from build123d import *

# Parameters (mm, degrees)
BOSS_EXTRUDE1_DEPTH = 1
SKETCH3_R           = 1.2
SKETCH3_R_2         = 3.05
CUT_EXTRUDE1_DEPTH  = 54.01311748


with BuildPart() as part:
    # Sketch1 → Boss-Extrude1 (new, symmetric)
    with BuildSketch(Plane(origin=(0, 0, 0), x_dir=(1, 0, 0), z_dir=(0, 1, 0))):
        with BuildLine():
            Line((22.2, 8.95), (22.2, -8.95))
            Line((22.2, -8.95), (40.625, -8.95))
            Line((40.625, -8.95), (40.625, -25.15))
            Line((40.625, -25.15), (22.879630679, -25.15))
            ThreePointArc((22.879630679, -25.15), (0, -34), (-22.879630679, -25.15))
            Line((-22.879630679, -25.15), (-40.625, -25.15))
            Line((-40.625, -25.15), (-40.625, -8.95))
            Line((-40.625, -8.95), (-22.2, -8.95))
            Line((-22.2, -8.95), (-22.2, 8.95))
            Line((-22.2, 8.95), (-40.625, 8.95))
            Line((-40.625, 8.95), (-40.625, 25.15))
            Line((-40.625, 25.15), (-22.879630679, 25.15))
            ThreePointArc((-22.879630679, 25.15), (0, 34), (22.879630679, 25.15))
            Line((22.879630679, 25.15), (40.625, 25.15))
            Line((40.625, 25.15), (40.625, 8.95))
            Line((40.625, 8.95), (22.2, 8.95))
        make_face()
    extrude(amount=BOSS_EXTRUDE1_DEPTH, both=True)

    # Sketch3 → Cut-Extrude1 (cut, through all)
    with BuildSketch(Plane(origin=(0, 1, 0), x_dir=(1, 0, 0), z_dir=(0, 1, 0))):
        with Locations(Location((-36.95, 17.05, 0), (0, 0, 270))):
            Circle(SKETCH3_R)
        with Locations(Location((-30, 17.05, 0), (0, 0, 270))):
            Circle(SKETCH3_R_2)
        with Locations(Location((-23.05, 17.05, 0), (0, 0, 270))):
            Circle(SKETCH3_R)
        with Locations(Location((23.05, 17.05, 0), (0, 0, 90))):
            Circle(SKETCH3_R)
        with Locations(Location((30, 17.05, 0), (0, 0, 90))):
            Circle(SKETCH3_R_2)
        with Locations(Location((36.95, 17.05, 0), (0, 0, 90))):
            Circle(SKETCH3_R)
        with Locations(Location((36.95, -17.05, 0), (0, 0, 270))):
            Circle(SKETCH3_R)
        with Locations(Location((30, -17.05, 0), (0, 0, 270))):
            Circle(SKETCH3_R_2)
        with Locations(Location((23.05, -17.05, 0), (0, 0, 270))):
            Circle(SKETCH3_R)
        with Locations(Location((-23.05, -17.05, 0), (0, 0, 90))):
            Circle(SKETCH3_R)
        with Locations(Location((-30, -17.05, 0), (0, 0, 90))):
            Circle(SKETCH3_R_2)
        with Locations(Location((-36.95, -17.05, 0), (0, 0, 90))):
            Circle(SKETCH3_R)
        with BuildLine():
            Line((1.55, 27.775), (1.55, -27.775))
            ThreePointArc((1.55, -27.775), (0, -29.325), (-1.55, -27.775))
            Line((-1.55, -27.775), (-1.55, 27.775))
            ThreePointArc((-1.55, 27.775), (0, 29.325), (1.55, 27.775))
        make_face()
        with BuildLine():
            Line((-18.5, 1.55), (-6.05, 1.55))
            ThreePointArc((-6.05, 1.55), (-4.5, 0), (-6.05, -1.55))
            Line((-6.05, -1.55), (-18.5, -1.55))
            ThreePointArc((-18.5, -1.55), (-20.05, 0), (-18.5, 1.55))
        make_face()
        with BuildLine():
            Line((6.05, 1.55), (18.5, 1.55))
            ThreePointArc((18.5, 1.55), (20.05, 0), (18.5, -1.55))
            Line((18.5, -1.55), (6.05, -1.55))
            ThreePointArc((6.05, -1.55), (4.5, 0), (6.05, 1.55))
        make_face()
        with BuildLine():
            Line((4.637438424, 6.738098576), (12.99447139, 25.238098576))
            ThreePointArc((12.99447139, 25.238098576), (15.045131543, 26.012561576), (15.819594543, 23.961901424))
            Line((15.819594543, 23.961901424), (7.462561576, 5.461901424))
            ThreePointArc((7.462561576, 5.461901424), (5.411901424, 4.687438424), (4.637438424, 6.738098576))
        make_face()
        with BuildLine():
            Line((4.687438424, 22.152061943), (7.73384453, 28.895904308))
            ThreePointArc((7.73384453, 28.895904308), (9.784504682, 29.670367308), (10.558967682, 27.619707155))
            Line((10.558967682, 27.619707155), (7.512561576, 20.875864791))
            ThreePointArc((7.512561576, 20.875864791), (5.461901424, 20.101401791), (4.687438424, 22.152061943))
        make_face()
        with BuildLine():
            Line((11.550411397, 6.738098576), (14.596817503, 13.481940941))
            ThreePointArc((14.596817503, 13.481940941), (16.647477655, 14.256403941), (17.421940655, 12.205743788))
            Line((17.421940655, 12.205743788), (14.375534549, 5.461901424))
            ThreePointArc((14.375534549, 5.461901424), (12.324874397, 4.687438424), (11.550411397, 6.738098576))
        make_face()
        with BuildLine():
            Line((-4.637438424, 6.738098576), (-12.99447139, 25.238098576))
            ThreePointArc((-12.99447139, 25.238098576), (-15.045131543, 26.012561576), (-15.819594543, 23.961901424))
            Line((-15.819594543, 23.961901424), (-7.462561576, 5.461901424))
            ThreePointArc((-7.462561576, 5.461901424), (-5.411901424, 4.687438424), (-4.637438424, 6.738098576))
        make_face()
        with BuildLine():
            Line((-4.687438424, 22.152061943), (-7.73384453, 28.895904308))
            ThreePointArc((-7.73384453, 28.895904308), (-9.784504682, 29.670367308), (-10.558967682, 27.619707155))
            Line((-10.558967682, 27.619707155), (-7.512561576, 20.875864791))
            ThreePointArc((-7.512561576, 20.875864791), (-5.461901424, 20.101401791), (-4.687438424, 22.152061943))
        make_face()
        with BuildLine():
            Line((-11.550411397, 6.738098576), (-14.596817503, 13.481940941))
            ThreePointArc((-14.596817503, 13.481940941), (-16.647477655, 14.256403941), (-17.421940655, 12.205743788))
            Line((-17.421940655, 12.205743788), (-14.375534549, 5.461901424))
            ThreePointArc((-14.375534549, 5.461901424), (-12.324874397, 4.687438424), (-11.550411397, 6.738098576))
        make_face()
        with BuildLine():
            Line((-4.637438424, -6.738098576), (-12.99447139, -25.238098576))
            ThreePointArc((-12.99447139, -25.238098576), (-15.045131543, -26.012561576), (-15.819594543, -23.961901424))
            Line((-15.819594543, -23.961901424), (-7.462561576, -5.461901424))
            ThreePointArc((-7.462561576, -5.461901424), (-5.411901424, -4.687438424), (-4.637438424, -6.738098576))
        make_face()
        with BuildLine():
            Line((-4.687438424, -22.152061943), (-7.73384453, -28.895904308))
            ThreePointArc((-7.73384453, -28.895904308), (-9.784504682, -29.670367308), (-10.558967682, -27.619707155))
            Line((-10.558967682, -27.619707155), (-7.512561576, -20.875864791))
            ThreePointArc((-7.512561576, -20.875864791), (-5.461901424, -20.101401791), (-4.687438424, -22.152061943))
        make_face()
        with BuildLine():
            Line((-11.550411397, -6.738098576), (-14.596817503, -13.481940941))
            ThreePointArc((-14.596817503, -13.481940941), (-16.647477655, -14.256403941), (-17.421940655, -12.205743788))
            Line((-17.421940655, -12.205743788), (-14.375534549, -5.461901424))
            ThreePointArc((-14.375534549, -5.461901424), (-12.324874397, -4.687438424), (-11.550411397, -6.738098576))
        make_face()
        with BuildLine():
            Line((4.637438424, -6.738098576), (12.99447139, -25.238098576))
            ThreePointArc((12.99447139, -25.238098576), (15.045131543, -26.012561576), (15.819594543, -23.961901424))
            Line((15.819594543, -23.961901424), (7.462561576, -5.461901424))
            ThreePointArc((7.462561576, -5.461901424), (5.411901424, -4.687438424), (4.637438424, -6.738098576))
        make_face()
        with BuildLine():
            Line((4.687438424, -22.152061943), (7.73384453, -28.895904308))
            ThreePointArc((7.73384453, -28.895904308), (9.784504682, -29.670367308), (10.558967682, -27.619707155))
            Line((10.558967682, -27.619707155), (7.512561576, -20.875864791))
            ThreePointArc((7.512561576, -20.875864791), (5.461901424, -20.101401791), (4.687438424, -22.152061943))
        make_face()
        with BuildLine():
            Line((11.550411397, -6.738098576), (14.596817503, -13.481940941))
            ThreePointArc((14.596817503, -13.481940941), (16.647477655, -14.256403941), (17.421940655, -12.205743788))
            Line((17.421940655, -12.205743788), (14.375534549, -5.461901424))
            ThreePointArc((14.375534549, -5.461901424), (12.324874397, -4.687438424), (11.550411397, -6.738098576))
        make_face()
    extrude(amount=-CUT_EXTRUDE1_DEPTH, mode=Mode.SUBTRACT)


solid = part.part
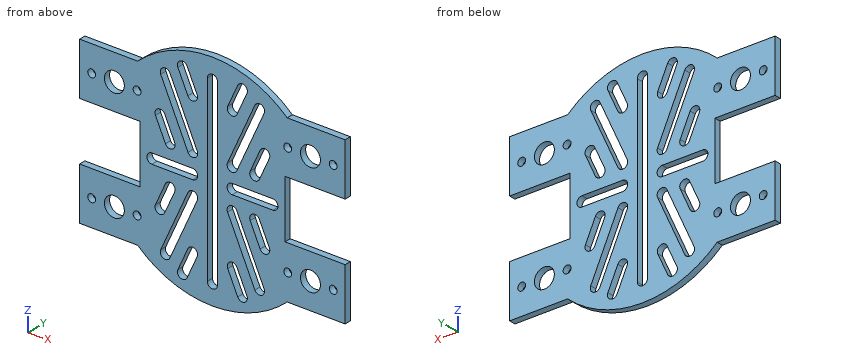
The listing builds one solid part. Answer for the finished solid, in the listing's coordinates (mm). Give positions to 0.01 mm unless a question says otherwise; leave off trailing zeros. Write each loop counter-clockwise with the first axis right and the second up, starting at its lowest first coordinate (ties: lowest second). Pieces come first, ordered by that corner, then holes. Notation, with made-up numbers: (80.5, -37) -> (127.5, -37) arc R20 ccw to (127.5, -4) -> close; hole circle Ø9 at (-25.5, 73). An arc over 180 degrees is marked (long way). Use a Markdown table: item, result.
(1) Section D-D, the plane y = 0.35 is taken. Give the number of separate pieces and of enclosed holes in the cut face, then the cut area to 3 significant figures.
Return value:
| item | result |
|---|---|
| separate pieces | 1 |
| enclosed holes | 27 |
| area | 3,030 mm2 |
(2) Find the intervals of material crossed by probe 1 along X at (y, z) = (0.45, 26); probe 2 along Z at (x, y) = (14, 0.65); probe 3 along X at (y, z) = (0.35, -9) (3 decimals), in increasing order. Write a range as from..to.
Return value:
| item | result |
|---|---|
| probe 1 | -21.91..-15.07, -13.74..-9.83, -6.43..-1.55, 1.55..6.43, 9.83..13.74, 15.07..21.91 |
| probe 2 | -30.98..-26.1, -19.93..-12.16, -4.95..-1.55, 1.55..4.95, 12.16..19.93, 26.1..30.98 |
| probe 3 | -40.625..-15.974, -12.572..-9.061, -5.659..-1.55, 1.55..5.659, 9.061..12.572, 15.974..40.625 |
(3) Section A-A, the plane x = -36.95 is taken. Determine the outline of the cut face in (y, z), then the cut area to 3 significant figures.
Return value:
| item | result |
|---|---|
| outline | (-1, -25.15) -> (1, -25.15) -> (1, -18.25) -> (-1, -18.25) -> close; (-1, -15.85) -> (1, -15.85) -> (1, -8.95) -> (-1, -8.95) -> close; (-1, 8.95) -> (1, 8.95) -> (1, 15.85) -> (-1, 15.85) -> close; (-1, 18.25) -> (1, 18.25) -> (1, 25.15) -> (-1, 25.15) -> close |
| area | 55.2 mm2 |
(4) Flat-ended cylindrical pins translate along their axes: P1, Ø0.6, axis at x = -11, y = -0.5, coming from the +Z side; P2, Ø1, axis at y = -0.5, z = -7.5, coming from the +X side; P3, Ø1, axis at x = -35, y = 0.5, coming from the -Z side. Find the tip coordinate at first contact, or state that the pin passes through.
Return value:
| item | result |
|---|---|
| P1 | z = 32.27 |
| P2 | x = 22.2 |
| P3 | z = -25.15 |
(5) Section B-B, the plane x = 0 is taken. Determine the outline of the cut face in (y, z) (3 decimals), then the cut area to 3 significant figures.
Return value:
| item | result |
|---|---|
| outline | (-1, -34) -> (1, -34) -> (1, -29.325) -> (-1, -29.325) -> close; (-1, 29.325) -> (1, 29.325) -> (1, 34) -> (-1, 34) -> close |
| area | 18.7 mm2 |
(6) Section C-C, the plane x = 30 is taken. Determine the outline of the cut face in (y, z), then the cut area to 3 significant figures.
Return value:
| item | result |
|---|---|
| outline | (-1, -25.15) -> (1, -25.15) -> (1, -20.1) -> (-1, -20.1) -> close; (-1, -14) -> (1, -14) -> (1, -8.95) -> (-1, -8.95) -> close; (-1, 8.95) -> (1, 8.95) -> (1, 14) -> (-1, 14) -> close; (-1, 20.1) -> (1, 20.1) -> (1, 25.15) -> (-1, 25.15) -> close |
| area | 40.4 mm2 |
